Work out the finished part from the listing and answer in its coordinate system (mm). A direction names the side the tool comes from. Give positions to 0.01 mm unless a question says otherwise; leave off trailing zeros. Loops run counter-clockwise (first coordinate to the right, second up) from the corner with the lowest first, then second, coordinate; pieces in that order, holes last. Notation, with made-up numbers: M 28.5,12 L 69.5,12 A26 ccw 69.5,41 Z; hole C 88.25,-13 d9. An arc over 180 degrees is marked long. Use a Markdown table: item, result.
```python
from build123d import *

# Parameters (mm, degrees)
F0_R     = 35
F0_R_2   = 25
F1_DEPTH = 15
F2_R     = 4.99999
F3_R     = 30.85
F3_R_2   = 25.79
F4_DEPTH = 7.065


# Not quite as in the source:
# - a fillet or chamfer is up to 0.001 mm smaller than in the source, because OpenCascade refuses the exact size


with BuildPart() as f1:
    # F0 (on Front) → F1 (new body, symmetric)
    with BuildSketch(Plane.XZ):
        Circle(F0_R)
        Circle(F0_R_2, mode=Mode.SUBTRACT)
    extrude(amount=F1_DEPTH, both=True)

    # F2 (radius 5 in the source; OpenCascade refuses exactly that, so slightly less here)
    f2_edges = [f1.edges().sort_by_distance(p)[0] for p in [
        (-35, -15, 0),
        (-25, -15, 0),
        (-35, 15, 0),
        (-25, 15, 0),
    ]]
    fillet(f2_edges, radius=F2_R)

    # F3 (on Front) → F4 (cut, symmetric)
    with BuildSketch(Plane.XZ):
        Circle(F3_R)
        Circle(F3_R_2, mode=Mode.SUBTRACT)
        Circle(F3_R_2)
    extrude(amount=F4_DEPTH, both=True, mode=Mode.SUBTRACT)


solid = f1.part
```
(1) Given P1, Ø4, axis at x = -15.5, y = -2, coming from the +Z side; P2, Ø6, axis at x = 16.5, y = -10, coming from the -Z side; P3, Ø1.5, axis at y = -3.5, z = 26, coming from the +X side, each flat-ended and moving along its own axis, determine where each tip first touches the part or whether it passes through.
Entries:
| item | result |
|---|---|
| P1 | stops at z = 32.29 |
| P2 | stops at z = -32.29 |
| P3 | stops at x = 24.24 |
(2) Consider probe 1 along Z at (x, y) = (0, 9); probe 2 along Y at (x, z) = (22.5, -20) (3 decimals); probe 3 along Z at (x, y) = (0, -0.75). Determine where each line is inside the solid, lowest interval first. Write a range as [from, to].
Entries:
| item | result |
|---|---|
| probe 1 | z = [-35, -25], [25, 35] |
| probe 2 | y = [-14.999, -7.065], [7.065, 14.999] |
| probe 3 | z = [-35, -30.85], [30.85, 35] |
(3) Which of the six approach directions +Z, -Z, +X, -X, +Y, -Y give full straight-line access (tool end or side, diameter ignored) to faces 3 (the cylindrical face through (23.846, 8.553, 7.509)), 4 (the flat face through (-0.1, -7.065, 25.3))?
Entries:
| item | result |
|---|---|
| face 3 | +Y, -Y |
| face 4 | none |
(4) The mould has two halves that part along X. Classify faces 1 (the cylindrical face through (-28, 0, -21)), 2 (the flat face through (-0.1, 7.065, 25.3)): released by +X, released by -X, zero draft, split by the parting line, or undercut.
Entries:
| item | result |
|---|---|
| face 1 | split by the parting line |
| face 2 | undercut |
(5) A cutting plane is placed at C-C (y = 5.5). Write down the section's boundary in (x, z), and give its area (3 significant figures).
Entries:
| item | result |
|---|---|
| outline | C 0,0 d70; hole C 0,0 d61.7 |
| area | 859 mm² |
